For this review, take the finished solid that the model builds, in its own axes (mm). A direction names the side the tool comes from. Coordinates: 2 decimals unless noted, no trailing zeros. Write each loop counter-clockwise with the first axis right and the second up, starting at its lowest first coordinate (ties: lowest second). Pieces come first, ordered by that corner, then holes.
```python
from build123d import *

# Parameters (mm, degrees)
EXTRUDE_1_DEPTH     = 7
SKETCH_2_R          = 6
CUT_EXTRUDE_1_DEPTH = 5.8
CUT_EXTRUDE_2_DEPTH = 0.2
FILLET_1_R          = 1
SKETCH_4_R          = 1.5
EXTRUDE_3_DEPTH     = 2.5
SKETCH_5_W          = 1.5
SKETCH_5_H          = 4.3
CUT_EXTRUDE_3_DEPTH = 2.5
SKETCH_6_W          = 3.174285876
SKETCH_6_H          = 3
CUT_EXTRUDE_4_DEPTH = 1


with BuildPart() as part:
    # Эскиз1 → Бобышка-Вытянуть1 (new body)
    with BuildSketch(Plane.XY):
        with BuildLine():
            Line((1.201755047, 83), (6.798244953, 83))
            ThreePointArc((6.798244953, 83), (7.648014096, 82.648014096), (8, 81.798244953))
            Line((8, 81.798244953), (8, 32.201755047))
            ThreePointArc((8, 32.201755047), (7.648014096, 31.351985904), (6.798244953, 31))
            Line((6.798244953, 31), (1.201755047, 31))
            ThreePointArc((1.201755047, 31), (0.351985904, 30.648014096), (0, 29.798244953))
            Line((0, 29.798244953), (0, 1.201755047))
            ThreePointArc((0, 1.201755047), (0.351985904, 0.351985904), (1.201755047, 0))
            Line((1.201755047, 0), (163.798244953, 0))
            ThreePointArc((163.798244953, 0), (164.648014096, 0.351985904), (165, 1.201755047))
            Line((165, 1.201755047), (165, 29.798244953))
            ThreePointArc((165, 29.798244953), (164.648014096, 30.648014096), (163.798244953, 31))
            Line((163.798244953, 31), (158.201755047, 31))
            ThreePointArc((158.201755047, 31), (157.351985904, 31.351985904), (157, 32.201755047))
            Line((157, 32.201755047), (157, 81.798244953))
            ThreePointArc((157, 81.798244953), (157.351985904, 82.648014096), (158.201755047, 83))
            Line((158.201755047, 83), (163.798244953, 83))
            ThreePointArc((163.798244953, 83), (164.648014096, 83.351985904), (165, 84.201755047))
            Line((165, 84.201755047), (165, 111.798244953))
            ThreePointArc((165, 111.798244953), (164.648014096, 112.648014096), (163.798244953, 113))
            Line((163.798244953, 113), (1.201755047, 113))
            ThreePointArc((1.201755047, 113), (0.351985904, 112.648014096), (0, 111.798244953))
            Line((0, 111.798244953), (0, 84.201755047))
            ThreePointArc((0, 84.201755047), (0.351985904, 83.351985904), (1.201755047, 83))
        make_face()
    extrude(amount=EXTRUDE_1_DEPTH)

    # Эскиз2 → Вырез-Вытянуть1 (cut)
    with BuildSketch(Plane(origin=(0, 0, 0), x_dir=(-1, 0, 0), z_dir=(0, 0, -1))):
        with BuildLine():
            Line((-161.798244953, 111), (-3.201755047, 111))
            ThreePointArc((-3.201755047, 111), (-2.351985904, 110.648014096), (-2, 109.798244953))
            Line((-2, 109.798244953), (-2, 86.201755047))
            ThreePointArc((-2, 86.201755047), (-2.351985904, 85.351985904), (-3.201755047, 85))
            Line((-3.201755047, 85), (-8.798244953, 85))
            ThreePointArc((-8.798244953, 85), (-9.648014096, 84.648014096), (-10, 83.798244953))
            Line((-10, 83.798244953), (-10, 30.201755047))
            ThreePointArc((-10, 30.201755047), (-9.648014096, 29.351985904), (-8.798244953, 29))
            Line((-8.798244953, 29), (-3.201755047, 29))
            ThreePointArc((-3.201755047, 29), (-2.351985904, 28.648014096), (-2, 27.798244953))
            Line((-2, 27.798244953), (-2, 3.201755047))
            ThreePointArc((-2, 3.201755047), (-2.351985904, 2.351985904), (-3.201755047, 2))
            Line((-3.201755047, 2), (-161.798244953, 2))
            ThreePointArc((-161.798244953, 2), (-162.648014096, 2.351985904), (-163, 3.201755047))
            Line((-163, 3.201755047), (-163, 27.798244953))
            ThreePointArc((-163, 27.798244953), (-162.648014096, 28.648014096), (-161.798244953, 29))
            Line((-161.798244953, 29), (-156.201755047, 29))
            ThreePointArc((-156.201755047, 29), (-155.351985904, 29.351985904), (-155, 30.201755047))
            Line((-155, 30.201755047), (-155, 70.5))
            Line((-155, 70.5), (-155, 74.8))
            Line((-155, 74.8), (-155, 83.798244953))
            ThreePointArc((-155, 83.798244953), (-155.351985904, 84.648014096), (-156.201755047, 85))
            Line((-156.201755047, 85), (-161.798244953, 85))
            ThreePointArc((-161.798244953, 85), (-162.648014096, 85.351985904), (-163, 86.201755047))
            Line((-163, 86.201755047), (-163, 109.798244953))
            ThreePointArc((-163, 109.798244953), (-162.648014096, 110.648014096), (-161.798244953, 111))
        make_face()
        with Locations((-82.5, 57)):
            Circle(SKETCH_2_R, mode=Mode.SUBTRACT)
    extrude(amount=-CUT_EXTRUDE_1_DEPTH, mode=Mode.SUBTRACT)

    # Эскиз3 → Вырез-Вытянуть2 (cut)
    # profile 1 of 2: a face of its own
    with BuildSketch(Plane(origin=(0, 0, 5.8), x_dir=(-1, 0, 0), z_dir=(0, 0, -1))):
        with BuildLine():
            Line((-120, 31), (-103, 31))
            ThreePointArc((-103, 31), (-102.292893219, 30.707106781), (-102, 30))
            Line((-102, 30), (-102, 19))
            ThreePointArc((-102, 19), (-102.292893219, 18.292893219), (-103, 18))
            Line((-103, 18), (-120, 18))
            ThreePointArc((-120, 18), (-120.707106781, 18.292893219), (-121, 19))
            Line((-121, 19), (-121, 30))
            ThreePointArc((-121, 30), (-120.707106781, 30.707106781), (-120, 31))
        make_face()
    # profile 2 of 2: a face of its own
    with BuildSketch(Plane(origin=(0, 0, 5.8), x_dir=(-1, 0, 0), z_dir=(0, 0, -1))):
        with BuildLine():
            Line((-52.1501229, 97.239252875), (-39.1501229, 97.239252875))
            ThreePointArc((-39.1501229, 97.239252875), (-38.443016119, 96.946359657), (-38.1501229, 96.239252875))
            Line((-38.1501229, 96.239252875), (-38.1501229, 83.239252875))
            ThreePointArc((-38.1501229, 83.239252875), (-38.443016119, 82.532146094), (-39.1501229, 82.239252875))
            Line((-39.1501229, 82.239252875), (-52.1501229, 82.239252875))
            ThreePointArc((-52.1501229, 82.239252875), (-52.857229681, 82.532146094), (-53.1501229, 83.239252875))
            Line((-53.1501229, 83.239252875), (-53.1501229, 96.239252875))
            ThreePointArc((-53.1501229, 96.239252875), (-52.857229681, 96.946359657), (-52.1501229, 97.239252875))
        make_face()
        Polygon((-41.403231286, 94.64375803), (-44.490035641, 94.64375803), (-48.784719961, 93.637191392), (-48.784719961, 92.630624755), (-44.490035641, 93.637191392), (-41.403231286, 93.637191392), align=None, mode=Mode.SUBTRACT)
        Polygon((-48.784719961, 91.774831443), (-44.490035641, 92.630624755), (-44.490035641, 91.774831443), (-48.784719961, 90.91903813), align=None, mode=Mode.SUBTRACT)
        Polygon((-48.784719961, 90.055112789), (-44.490035641, 90.910906102), (-44.490035641, 90.055112789), (-48.784719961, 89.067866896), align=None, mode=Mode.SUBTRACT)
        Polygon((-48.784719961, 88.216527408), (-44.490035641, 89.067866896), (-41.403231286, 89.067866896), (-41.403231286, 88.316883581), (-44.341167482, 88.316883581), (-48.784719961, 87.436033812), align=None, mode=Mode.SUBTRACT)
        Polygon((-48.609605566, 93.888102843), (-44.858812452, 94.806018458), (-44.858812452, 95.913847648), (-46.734209009, 95.170019477), (-48.609605566, 95.739760204), align=None, mode=Mode.SUBTRACT)
        Polygon((-48.609605566, 87.006809767), (-44.858812452, 87.715709289), (-44.858812452, 86.328076183), (-46.734209009, 86.674984459), (-48.609605566, 85.770006347), align=None, mode=Mode.SUBTRACT)
    extrude(amount=-CUT_EXTRUDE_2_DEPTH, mode=Mode.SUBTRACT)

    # Скругление1
    fillet_1_edges = [part.edges().sort_by_distance(p)[0] for p in [
        (155, 57, 5.8),
        (155.351985904, 84.648014096, 5.8),
        (159, 85, 5.8),
        (162.648014096, 85.351985904, 5.8),
        (163, 98, 5.8),
        (162.648014096, 110.648014096, 5.8),
        (82.5, 111, 5.8),
        (2.351985904, 110.648014096, 5.8),
        (2, 98, 5.8),
        (2.351985904, 85.351985904, 5.8),
        (6, 85, 5.8),
        (9.648014096, 84.648014096, 5.8),
        (10, 57, 5.8),
        (9.648014096, 29.351985904, 5.8),
        (6, 29, 5.8),
        (2.351985904, 28.648014096, 5.8),
        (2, 15.5, 5.8),
        (2.351985904, 2.351985904, 5.8),
        (82.5, 2, 5.8),
        (162.648014096, 2.351985904, 5.8),
        (163, 15.5, 5.8),
        (162.648014096, 28.648014096, 5.8),
        (159, 29, 5.8),
        (155.351985904, 29.351985904, 5.8),
    ]]
    fillet(fillet_1_edges, radius=FILLET_1_R)

    # Эскиз4 → Бобышка-Вытянуть3 (add)
    # profile 1 of 2: a face of its own
    with BuildSketch(Plane(origin=(0, 0, 0), x_dir=(-1, 0, 0), z_dir=(0, 0, -1))):
        with BuildLine():
            Line((-157, 73), (-163.5, 73))
            ThreePointArc((-163.5, 73), (-164.207106781, 72.707106781), (-164.5, 72))
            Line((-164.5, 72), (-164.5, 41))
            ThreePointArc((-164.5, 41), (-164.207106781, 40.292893219), (-163.5, 40))
            Line((-163.5, 40), (-157, 40))
            Line((-157, 40), (-157, 73))
        make_face()
        with Locations((-161.7, 47)):
            Circle(SKETCH_4_R, mode=Mode.SUBTRACT)
        with Locations((-161.7, 65)):
            Circle(SKETCH_4_R, mode=Mode.SUBTRACT)
    # profile 2 of 2: a face of its own
    with BuildSketch(Plane(origin=(0, 0, 0), x_dir=(-1, 0, 0), z_dir=(0, 0, -1))):
        with BuildLine():
            Line((-1.5, 73), (-8, 73))
            Line((-8, 73), (-8, 40))
            Line((-8, 40), (-1.5, 40))
            ThreePointArc((-1.5, 40), (-0.792893219, 40.292893219), (-0.5, 41))
            Line((-0.5, 41), (-0.5, 72))
            ThreePointArc((-0.5, 72), (-0.792893219, 72.707106781), (-1.5, 73))
        make_face()
        with Locations((-3.3, 47)):
            Circle(SKETCH_4_R, mode=Mode.SUBTRACT)
        with Locations((-3.3, 65)):
            Circle(SKETCH_4_R, mode=Mode.SUBTRACT)
    extrude(amount=-EXTRUDE_3_DEPTH)

    # Эскиз5 → Вырез-Вытянуть3 (cut)
    with BuildSketch(Plane(origin=(0, 0, 0), x_dir=(-1, 0, 0), z_dir=(0, 0, -1))):
        with Locations((-155.75, 72.65)):
            Rectangle(SKETCH_5_W, SKETCH_5_H)
    extrude(amount=-CUT_EXTRUDE_3_DEPTH, mode=Mode.SUBTRACT)

    # Эскиз6 → Вырез-Вытянуть4 (cut)
    with BuildSketch(Plane(origin=(0, 0, 0), x_dir=(-1, 0, 0), z_dir=(0, 0, -1))):
        with Locations((-156.587142938, 81.5)):
            Rectangle(SKETCH_6_W, SKETCH_6_H)
    extrude(amount=-CUT_EXTRUDE_4_DEPTH, mode=Mode.SUBTRACT)


solid = part.part
```
1) Consider section C-C (y = 68.5). Give the boundary of the cut face in (x, z).
2) Tool access review of faces 1 (the face through (161, 57, 2.5)), 2 (the face through (0, 16, 3)), 3 (the face through (163, 15, 2)): name each direction out of +Z, -Z, +X, -X, +Y, -Y from which nothing blocks a thin tool from reaching the whole face with its end or side.
3) Clearance check with flat-ended pins moving along their axes: P1, Ø0.6, axis at x = 46.5, y = 94.5, coming from the -Z side; P2, Ø0.9, axis at x = 156.5, y = 81.5, coming from the -Z side; P3, Ø1.2, axis at y = 73, z = 1, coming from the -X side. State where each tip first meets the part, or that it passes through.
4) The part is to be moulded in two halves that separate along Y. For faces 4 (the face through (82, 57, 0)), 5 (the face through (84, 113, 3)), 6 (the face through (2, 16, 2)), say which applies: pulls with the +Y half, pulls with the -Y half, needs draft (parallel to the pull), parting line crosses it, or undercut.
5) Consider section A-A (y = 57). Give the boundary of the cut face in (x, z), then the cut area to 3 significant figures.
6) Consider section B-B (x = 136). Give the boundary of the cut face in (y, z).
7) For L1, parallel to Y at x = 98.5, z = 3.5; L2, parallel to Y at x = 7, z = 6.25; L3, parallel to X at y = 37.5, z = 4.5, list the stretches that pass through material, from the lowest coordinate up.
Results:
1. outline: (0.5, 0) - (10, 0) - (10, 4.8) arc R1 cw to (11, 5.8) - (154, 5.8) arc R1 cw to (155, 4.8) - (155, 0) - (164.5, 0) - (164.5, 2.5) - (157, 2.5) - (157, 7) - (8, 7) - (8, 2.5) - (0.5, 2.5) - close
2. face 1: +Z, +X
2. face 2: +Z, -Z, -X, +Y, -Y
2. face 3: -Z
3. P1: stops at z = 5.8
3. P2: stops at z = 1
3. P3: stops at x = 0.58
4. face 4: needs draft
4. face 5: pulls with the +Y half
4. face 6: undercut
5. outline: (0.5, 0) - (10, 0) - (10, 4.8) arc R1 cw to (11, 5.8) - (76.5, 5.8) - (76.5, 0) - (88.5, 0) - (88.5, 5.8) - (154, 5.8) arc R1 cw to (155, 4.8) - (155, 0) - (164.5, 0) - (164.5, 2.5) - (157, 2.5) - (157, 7) - (8, 7) - (8, 2.5) - (0.5, 2.5) - close
5. area: 310 mm2
6. outline: (0, 0) - (2, 0) - (2, 4.8) arc R1 cw to (3, 5.8) - (110, 5.8) arc R1 cw to (111, 4.8) - (111, 0) - (113, 0) - (113, 7) - (0, 7) - close
7. L1: y = 0 to 2, 111 to 113
7. L2: y = 0 to 31.02, 82.98 to 113
7. L3: x = 8 to 10, 155 to 157
